```python
from build123d import *

# Parameters (mm, degrees)
F0_W        = 22.621599026
F0_H        = 39.9586446583
F1_DEPTH    = 25.4
F2_W        = 9.6419928595
F2_H        = 15.4364593327
F3_DEPTH    = 25.401
F4_T1_DEPTH = 25.4
F5_W        = 5.1918416284
F5_H        = 8.622167632
F6_DEPTH    = 25.401
F8_DEPTH    = 0.254
F9_DEPTH    = 5.08


# Not quite as in the source:
# - a fillet or chamfer that OpenCascade refuses, or shapes differently, is made with other operations: its cross-section is extruded or revolved along the edge and cut away or added


with BuildPart() as f1:
    # F0 (on Front) → F1 (new body)
    with BuildSketch(Plane.XZ):
        with Locations((0.185423065, 19.9793223292)):
            Rectangle(F0_W, F0_H)
    extrude(amount=F1_DEPTH)

    # F2 (on face) → F3 (cut, through all)
    with BuildSketch(Plane.XZ.offset(25.4)):
        with Locations((0.1854221337, 32.240414992)):
            Rectangle(F2_W, F2_H)
    extrude(amount=-F3_DEPTH, mode=Mode.SUBTRACT)

    # F4: fillet of radius 5.08 on 2 edges, made by hand

    # F4_s2 → F4_t1 (join)
    with BuildSketch(Plane.XZ):
        with BuildLine():
            ThreePointArc((-4.6355742961, 29.6021853256), (-3.1476767445, 26.0100828772), (0.4444257039, 24.5221853256))
            Line((0.4444257039, 24.5221853256), (-4.6355742961, 24.5221853256))
            Line((-4.6355742961, 24.5221853256), (-4.6355742961, 29.6021853256))
        make_face()
        with BuildLine():
            ThreePointArc((-0.0735814366, 24.5221853256), (3.5185210119, 26.0100828772), (5.0064185634, 29.6021853256))
            Line((5.0064185634, 29.6021853256), (5.0064185634, 24.5221853256))
            Line((5.0064185634, 24.5221853256), (-0.0735814366, 24.5221853256))
        make_face()
    extrude(amount=F4_T1_DEPTH)

    # F5 (on face) → F6 (cut, through all)
    with BuildSketch(Plane.XZ.offset(25.4)):
        with Locations((8.9003017638, 4.311083816)):
            Rectangle(F5_W, F5_H)
    extrude(amount=-F6_DEPTH, mode=Mode.SUBTRACT)

    # F7 (on Top) → F8 (join)
    with BuildSketch(Plane.XY):
        with BuildLine():
            Line((6.3043809496, 0), (-10.9399538487, 0))
            Line((-10.9399538487, 0), (-10.9399538487, -45.7067526877))
            ThreePointArc((-10.9399538487, -45.7067526877), (0.463556964, -57.1102635004), (11.8670677766, -45.7067526877))
            Line((11.8670677766, -45.7067526877), (11.8670677766, -33.1019833684))
            Line((11.8670677766, -33.1019833684), (6.3043809496, -33.1019833684))
            Line((6.3043809496, -33.1019833684), (6.3043809496, -25.4))
            Line((6.3043809496, -25.4), (6.3043809496, 0))
        make_face()
    extrude(amount=F8_DEPTH)

    # F9 (add): a face of the model
    f9_faces = [f1.faces().sort_by_distance(p)[0] for p in [
        (-0.1279092973, -40.8893319154, 0.254),
    ]]
    extrude(f9_faces, amount=F9_DEPTH)


solid = f1.part
```
Source: CAD feature listing. Evaluate the final solid. Frame: model axes, mm. A direction names the side the tool comes from. Round coordinates to 2 decimals unless told otherwise and drop trailing zeros. Write each loop counter-clockwise with the first axis right and the second up, starting at its lowest first coordinate (ties: lowest second). Pieces come first, ordered by that corner, then holes. Notation, with made-up numbers: M 46,-1.75 L 103,-1.75 A12 cw 103,21.25 Z; hole C 50,-28 d8. An arc over 180 degrees is marked long. Answer as a JSON object with one key per item and string values. Group by question number.
(1) Section query C-C on y = -2.5. Output: boundary loops of the cut face in (x, z).
(2) Section query D-D on x = 7.5. Output: boundary loops of the cut face in (y, z).
(3) Reachability of faces 1 (the flat face through (9, -13, 8.622)), 2 (the flat face through (-10.94, -35, 3)), 3 (the cylindrical face through (3.57, -12.52, 26.06)), 4 (the flat face through (0, -41, 5.334)) from +Z, -Z, +X, -X, +Y, -Y: full face, straight path, thin tool, end or side. Return the list, or none.
(4) Ray query, line 1 (X direction, y = -4, z = 33); line 2 (Y direction, x = -9, z = 25); line 3 (Z direction, x = -2.5, y = -33). Return the intervals inside material, ascending. Write a range as [from, to].
(5) First-contact query: pin 1 (1.6 mm diameter, centred on x = 9.5, y = -9.5, fed in from -Z); pin 2 (6 mm diameter, centred on y = -33.5, z = 1.5, fed in from -X); pin 3 (2 mm diameter, centred on y = -10, z = 30.5, fed in from +X); pin 4 (10 mm diameter, centred on x = -4.5, z = 8.5, fed in from +Y). Flat tips, straight axial feed; report the tip coordinate or a pass-through.
(6) Section query A-A on z = 37.5. Output: boundary loops of the cut face in (x, y).
(7) Section query B-B on z = 4.5. Output: boundary loops of the cut face in (x, y), then the cut area to 3 significant figures.
(8) Mould query, pull axis X, two halves, no side actions, for faces 5 (the cylindrical face through (-3.275, -12.522, 26.142)), 6 (the flat face through (9, -33.102, 3)), 7 (the cylindrical face through (0.213, -57.108, 2.63)). Classes: +X half, -X half, draft (parallel to the pull), parting line (faces both ways), or undercut.
Computed values:
{
 "1": {"outline": "M -11.13,0 L 6.3,0 L 6.3,8.62 L 11.5,8.62 L 11.5,39.96 L 5.01,39.96 L 5.01,29.6 A5.08 cw 0.19,24.53 A5.08 cw -4.64,29.6 L -4.64,39.96 L -11.13,39.96 Z"},
 "2": {"outline": "M -54.68,0 L -33.1,0 L -33.1,5.33 L -54.68,5.33 Z; M -25.4,8.62 L 0,8.62 L 0,39.96 L -25.4,39.96 Z"},
 "3": {"face 1": "-Z, +X, +Y, -Y", "face 2": "+Z, -Z, -X, -Y", "face 3": "+Z, +Y, -Y", "face 4": "+Z, +X, -X, -Y"},
 "4": {"line 1": "[-11.13, -4.64], [5.01, 11.5]", "line 2": "[-25.4, 0]", "line 3": "[0, 5.33]"},
 "5": {"pin 1": "z = 8.62", "pin 2": "x = -10.94", "pin 3": "x = 11.5", "pin 4": "y = 0"},
 "6": {"outline": "M -11.13,-25.4 L -4.64,-25.4 L -4.64,0 L -11.13,0 Z; M 5.01,-25.4 L 11.5,-25.4 L 11.5,0 L 5.01,0 Z"},
 "7": {"outline": "M -11.13,-25.4 L -10.94,-25.4 L -10.94,-45.71 A11.4 ccw 11.87,-45.71 L 11.87,-33.1 L 6.3,-33.1 L 6.3,0 L -11.13,0 Z", "area": "1,070 mm^2"},
 "8": {"face 5": "undercut", "face 6": "draft", "face 7": "parting line"}
}
